Input: part model. Units: mm. Frame: model coordinates. Face numbers are marked on the shaded views. A direction names the side the tool comes from. Coordinates: 2 decimals unless noted, no trailing zeros. Write each loop counter-clockwise with the first axis right and the second up, starting at its lowest first coordinate (ties: lowest second). Pieces come first, ordered by that corner, then holes.
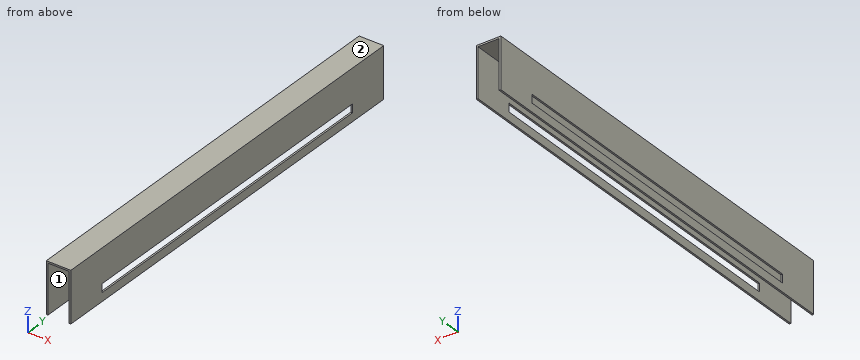
from build123d import *

# Parameters (mm, degrees)
BOSS_EXTRUDE1_DEPTH     = 500
CUT_EXTRUDE1_DEPTH      = 503.06174919
CUT_EXTRUDE1_DEPTH_BACK = 503.06174919
SKETCH2_W               = 10
SKETCH2_H               = 400


with BuildPart() as part:
    # Sketch1 → Boss-Extrude1 (new body)
    with BuildSketch(Plane(origin=(0, 0, 0), x_dir=(1, 0, 0), z_dir=(0, 1, 0))):
        Polygon((-25, -33), (-25, 25), (-27, 25), (-27, -35), (2, -35), (2, 25), (0, 25), (0, -33), align=None)
    extrude(amount=BOSS_EXTRUDE1_DEPTH)

    # Sketch2 → Cut-Extrude1 (cut, two sides: drawn at the far end of the back side and taken through both)
    with BuildSketch(Plane(origin=(2, 0, 0), x_dir=(0, 0, -1), z_dir=(1, 0, 0)).offset(-CUT_EXTRUDE1_DEPTH_BACK)):
        with Locations((10, 250)):
            Rectangle(SKETCH2_W, SKETCH2_H)
    extrude(amount=CUT_EXTRUDE1_DEPTH + CUT_EXTRUDE1_DEPTH_BACK, mode=Mode.SUBTRACT)


solid = part.part
Item 1: Material intervals for line 1 (X direction, y = 465.5, z = 0); line 2 (Z direction, x = -16.75, y = 362), sorted ascending.
Item 2: Pin query (flat end, axial travel): pin 1 Ø12 at (x, y) = (-7.5, 72.5) entering from -Z; pin 2 Ø2 at (x, z) = (0.5, -8.5) entering from -Y; pin 3 Ø3 at (x, z) = (-23, -0.5) entering from +Y. Return the tip coordinate at first contact, or that it passes through.
Item 3: Section query A-A, the plane y = 199. Return loops of the section in (x, z).
Item 4: Section query B-B, the plane z = 7. Return loops of the section in (x, y).
Item 5: Section query D-D, the plane x = -17.5. Return loops of the section in (y, z), then the cut area to 3 significant figures.
Item 6: Access query for the marked faces 1 and 2. Directions: +Z, -Z, +X, -X, +Y, -Y. A direction counts if a zero-diameter tool reaches every point of the face in a straight line with its end or side. Return the directions, or none.
Item 7: Section query C-C, the plane y = 36. Return loops of the section in (x, z), then the cut area to 3 significant figures.
The answers:
1. line 1: x = -27 to -25, 0 to 2
1. line 2: z = 33 to 35
2. pin 1: stops at z = 33
2. pin 2: stops at y = 0
2. pin 3: passes through
3. outline: (-27, -25) - (-25, -25) - (-25, -15) - (-27, -15) - close; (-27, -5) - (-25, -5) - (-25, 33) - (0, 33) - (0, -5) - (2, -5) - (2, 35) - (-27, 35) - close; (0, -25) - (2, -25) - (2, -15) - (0, -15) - close
4. outline: (-27, 0) - (-25, 0) - (-25, 500) - (-27, 500) - close; (0, 0) - (2, 0) - (2, 500) - (0, 500) - close
5. outline: (0, 33) - (500, 33) - (500, 35) - (0, 35) - close
5. area: 1,000 mm2
6. face 1: -Z, +Y, -Y
6. face 2: +Z, +X, -X, +Y, -Y
7. outline: (-27, -25) - (-25, -25) - (-25, 33) - (0, 33) - (0, -25) - (2, -25) - (2, 35) - (-27, 35) - close
7. area: 290 mm2
